```python
from build123d import *

# Parameters (mm, degrees)
SKETCH1_W           = 20
SKETCH1_H           = 4
BOSS_EXTRUDE1_DEPTH = 160
CUT_EXTRUDE1_REACH  = 163.295
SKETCH2_R           = 1.4


with BuildPart() as part:
    # Sketch1 → Boss-Extrude1 (new body)
    with BuildSketch(Plane(origin=(0, 0, 0), x_dir=(1, 0, 0), z_dir=(0, 1, 0))):
        with Locations((-10, -2)):
            Rectangle(SKETCH1_W, SKETCH1_H)
    extrude(amount=BOSS_EXTRUDE1_DEPTH)

    # Sketch2 → Cut-Extrude1 (cut, up to next)
    with BuildSketch(Plane(origin=(0, 0, 0), x_dir=(-1, 0, 0), z_dir=(0, -1, 0)), mode=Mode.PRIVATE) as cut_extrude1_sk1:
        with Locations(Location((18, -2, 0), (0, 0, 90))):
            Circle(SKETCH2_R)
    cut_extrude1_tool1 = extrude(cut_extrude1_sk1.sketch, amount=-CUT_EXTRUDE1_REACH, mode=Mode.PRIVATE) & part.part
    # Sketch2 → Cut-Extrude1 (cut, up to next)
    with BuildSketch(Plane(origin=(0, 0, 0), x_dir=(-1, 0, 0), z_dir=(0, -1, 0)), mode=Mode.PRIVATE) as cut_extrude1_sk2:
        with Locations(Location((2, -2, 0), (0, 0, 90))):
            Circle(SKETCH2_R)
    cut_extrude1_tool2 = extrude(cut_extrude1_sk2.sketch, amount=-CUT_EXTRUDE1_REACH, mode=Mode.PRIVATE) & part.part
    add(cut_extrude1_tool1.solids().sort_by_distance((-18, 0, 2))[0], mode=Mode.SUBTRACT)
    add(cut_extrude1_tool2.solids().sort_by_distance((-2, 0, 2))[0], mode=Mode.SUBTRACT)


solid = part.part
```
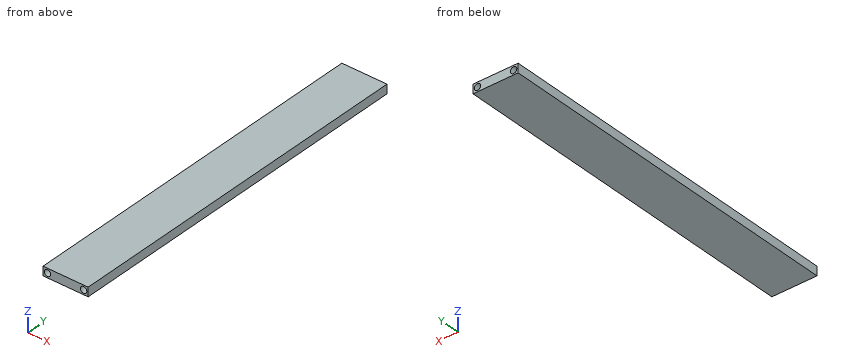
CAD build for the part. Positions are in the model's coordinates, mm. Round coordinates to 2 decimals unless told otherwise and drop trailing zeros. Write each loop counter-clockwise with the first axis right and the second up, starting at its lowest first coordinate (ties: lowest second). Pieces come first, ordered by that corner, then holes. Notation, with made-up numbers: (71, 34) - (80, 34) arc R35 ccw to (80, 68) - close; hole circle Ø5 at (10, 40). An arc over 180 degrees is marked (long way). Return JSON: item names as keys, results as strings. Group by question number.
Item 1: Band-saw the part on C-C on y = 50. List the corners of the cut face in (x, z), plus the area to 3 significant figures.
Item 2: Band-saw the part on A-A on x = -18. List the corners of the cut face in (y, z), plus the area to 3 significant figures.
Item 3: Band-saw the part on B-B on z = 2.8. List the corners of the cut face in (x, y).
Item 4: Probe probe 1 along X at (y, z) = (104.5, 2); probe 2 along X at (y, z) = (46, 2.95); probe 3 along Z at (x, y) = (-17.5, 105.5). List the from-to ranges inside material, lowest first.
Resolved:
{
 "1": {"outline": "(-20, 0) - (0, 0) - (0, 4) - (-20, 4) - close; hole circle Ø2.8 at (-18, 2); hole circle Ø2.8 at (-2, 2)", "area": "67.7 mm²"},
 "2": {"outline": "(0, 0) - (160, 0) - (160, 0.6) - (0, 0.6) - close; (0, 3.4) - (160, 3.4) - (160, 4) - (0, 4) - close", "area": "192 mm²"},
 "3": {"outline": "(-20, 0) - (-19.15, 0) - (-19.15, 160) - (-20, 160) - close; (-16.85, 0) - (-3.15, 0) - (-3.15, 160) - (-16.85, 160) - close; (-0.85, 0) - (0, 0) - (0, 160) - (-0.85, 160) - close"},
 "4": {"probe 1": "x = -20 to -19.4, -16.6 to -3.4, -0.6 to 0", "probe 2": "x = -20 to -19.03, -16.97 to -3.03, -0.97 to 0", "probe 3": "z = 0 to 0.69, 3.31 to 4"}
}
